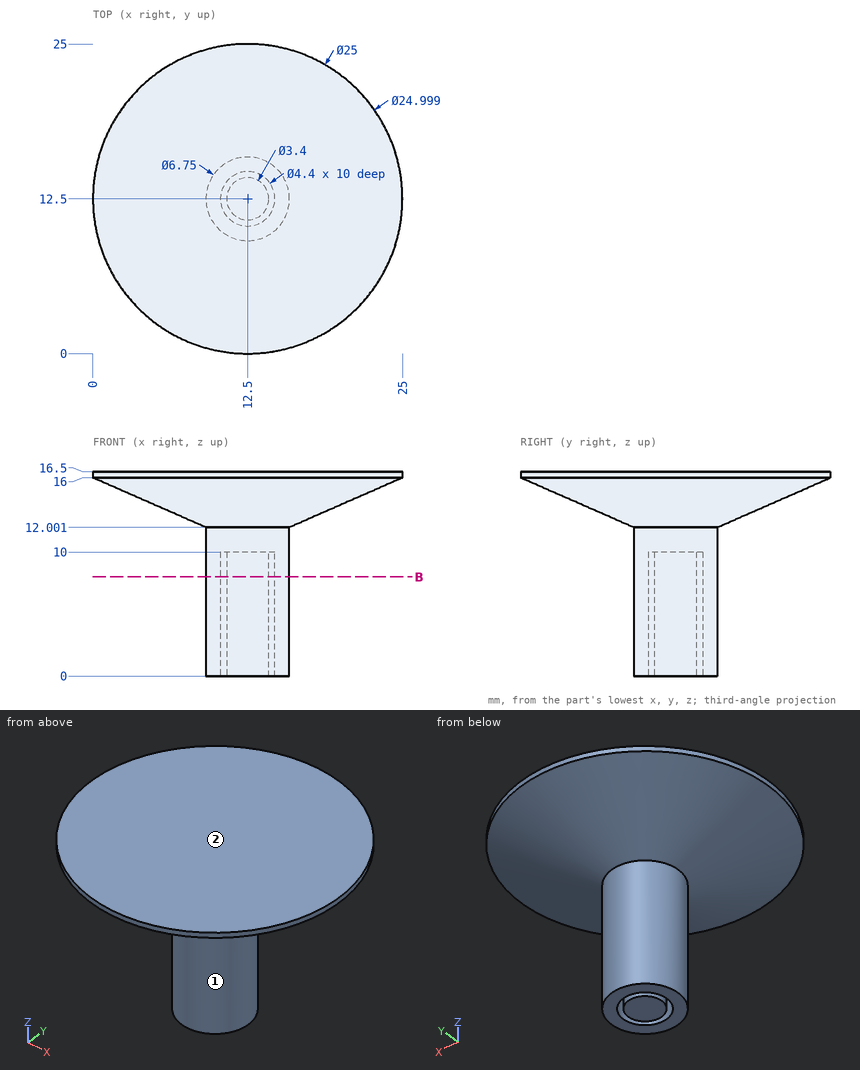
Study the drawing (mm; zero at the part's minimum x, y, z) and answer. A direction names the side the tool comes from. Round coordinates to 2 decimals unless told otherwise and drop trailing zeros. Write each question's results on one line, items separated by ' | '. Start each with the question number.
1. Find the intervals of material crossed by probe 1 along Y at (x, z) = (12.5, 5.25) (1 decimal); probe 2 along Y at (x, z) = (13, 4) (1 decimal); probe 3 along Z at (x, y) = (18.75, 2), in increasing order. Write a range as from..to.
2. A tool of negligible diameter and unlimited length cuts with its end or side. For the marked faces 1 and 2, from which of +Z, -Z, +X, -X, +Y, -Y can it reach the whole face along a straight path? Write none if from no direction.
3. Section B-B (z = 8) is taken. State how many separate pieces and enclosed holes the cut face has.
4. Given pin 1 Ø6 at (x, y) = (17, 2.5) entering from -Z; pin 2 Ø3 at (x, z) = (12.5, 9.5) entering from -Y (1 decimal); pin 3 Ø8 at (y, z) = (15, 1.5) entering from -X (1 decimal), each flat-ended and moving along its own axis, determine where each tip first touches the part or whether it passes through.
Evaluation:
1) probe 1: y = 9.1..10.3, 10.8..14.2, 14.7..15.9 | probe 2: y = 9.2..10.4, 10.9..14.1, 14.6..15.8 | probe 3: z = 15.88..16.5
2) face 1: -Z | face 2: +Z, +X, -X, +Y, -Y
3) separate pieces: 2 | enclosed holes: 1
4) pin 1: stops at z = 14.01 | pin 2: stops at y = 9.1 | pin 3: stops at x = 9.1
